Input: part model. Units: mm. Frame: model coordinates. Coordinates: 2 decimals unless noted, no trailing zeros. Loops run counter-clockwise (first coordinate to the right, second up) from the corner with the lowest first, then second, coordinate; pieces in that order, holes last. Notation, with made-up numbers: (-3.75, 89.5) - (26.25, 89.5) arc R35 cw to (26.25, 124.5) - close; hole circle Ø1 at (5, -7). An arc over 180 degrees is marked (long way). Use a Markdown table: item, result. Add a question column.
1. Ray query, L1, parallel to Z at x = 69.5, y = 2.5; L2, parallel to Y at x = 14.25, z = -4; L3, parallel to Z at x = 6, y = 1.5. Return the intervals inside material, ascending. Write a range as [from, to].
2. Section query B-B on y = 2.5. Return the cut outline in (x, z).
3. Section query C-C on z = -4. Return the cut outline in (x, y), then the cut area to 3 significant figures.
4. Contact query for a flat-ended pin moving along its axis: P1, Ø2, axis at y = 2.5, z = -36, coming from the -X side. Output: stop coordinate, or through.
5. Section query A-A on x = 71.5. Return the cut outline in (y, z), then the cut area to 3 significant figures.
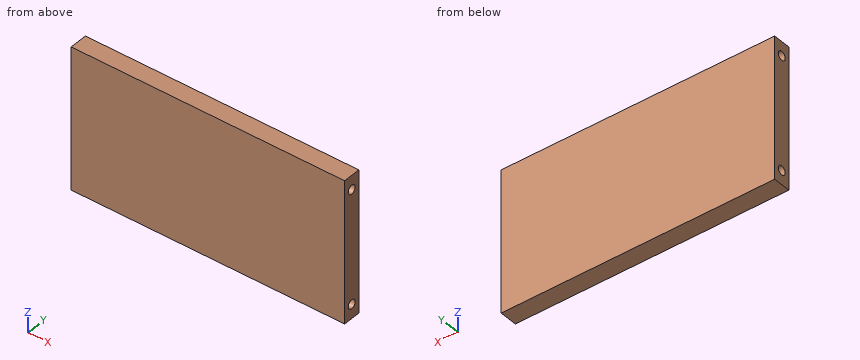
Autodesk Inventor part; units mm, degrees
ref_plane "YZ Plane" through (0, 0, 0) normal (1, 0, 0) x (0, 1, 0)
ref_plane "XZ Plane" through (0, 0, 0) normal (0, 1, 0) x (-1, 0, 0)
ref_plane "XY Plane" through (0, 0, 0) normal (0, 0, 1) x (1, 0, 0)
sketch "スケッチ2" plane through (0, 0, 0) normal (0, 1, 0) x (-1, 0, 0)
  line L0 (0, 0) -> (-77, 0)
  line L1 (-77, 0) -> (-77, -40)
  line L2 (-77, -40) -> (0, -40)
  line L3 (0, -40) -> (0, 0)
  dimension "d0" = 77
  dimension "d1" = 40
extrude "押し出し1" add sketch "スケッチ2" along normal blind 5
sketch "スケッチ4" plane through (0, 0, -40) normal (-1, 0, 0) x (0, 0, 1)
  line L0 (0, 0) -> (0, 5) construction
  line L1 (0, 2.5) -> (40, 2.5) construction
  line L2 (40, 0) -> (40, 5) construction
  point P0 (4, 2.5)
  point P1 (36, 2.5)
  dimension "d4" = 4
  dimension "d5" = 4
hole "穴1" at (0, 2.5, -36) at (0, 2.5, -4) direction (1, 0, 0) diameter 2.459 depth 20
sketch "スケッチ5" plane through (77, 0, 0) normal (1, 0, 0) x (0, 0, -1)
  line L0 (0, 0) -> (0, 5) construction
  line L1 (0, 2.5) -> (39.9198, 2.5) construction
  circle A0 centre (4, 2.5) radius 1.2295 construction
  circle A1 centre (36, 2.5) radius 1.2295
hole "穴2" at (77, 2.5, -4) at (77, 2.5, -36) direction (-1, 0, 0) diameter 2.459 depth 20
properties part number "shoulder1_verticval_plate"
Resolved:
| question | item | result |
|---|---|---|
| 1 | L1 | [-40, -37.23], [-34.77, -5.23], [-2.77, 0] |
| 1 | L2 | [0, 1.27], [3.73, 5] |
| 1 | L3 | [-40, -36.72], [-35.28, -4.72], [-3.28, 0] |
| 2 | outline | (0, -40) - (77, -40) - (77, -37.23) - (57, -37.23) - (57, -34.77) - (77, -34.77) - (77, -5.23) - (57, -5.23) - (57, -2.77) - (77, -2.77) - (77, 0) - (0, 0) - (0, -2.77) - (20, -2.77) - (20, -5.23) - (0, -5.23) - (0, -34.77) - (20, -34.77) - (20, -37.23) - (0, -37.23) - close |
| 3 | outline | (0, 0) - (77, 0) - (77, 1.27) - (57, 1.27) - (57, 3.73) - (77, 3.73) - (77, 5) - (0, 5) - (0, 3.73) - (20, 3.73) - (20, 1.27) - (0, 1.27) - close |
| 3 | area | 287 mm² |
| 4 | P1 | x = 20 |
| 5 | outline | (0, -40) - (5, -40) - (5, 0) - (0, 0) - close; hole circle Ø2.46 at (2.5, -36); hole circle Ø2.46 at (2.5, -4) |
| 5 | area | 191 mm² |
